```python
from build123d import *

# Parameters (mm, degrees)
SKETCH_1_R          = 5.25
EXTRUDE_1_DEPTH     = 5
CHAMFER_1_SIZE      = 0.4
SKETCH_2_R          = 1.2
CUT_EXTRUDE_1_DEPTH = 2.5
SKETCH_3_R          = 0.75
EXTRUDE_2_DEPTH     = 0.2
SKETCH_4_R          = 0.6
EXTRUDE_3_DEPTH     = 0.2
SKETCH_5_R          = 0.5
EXTRUDE_4_DEPTH     = 5.5
FILLET_1_R          = 0.1
SKETCH_6_R          = 2.5
EXTRUDE_5_DEPTH     = 1.7
EXTRUDE_6_DEPTH     = 1
SKETCH_8_R          = 0.7
CUT_EXTRUDE_2_DEPTH = 1
SKETCH_9_R          = 1.5
EXTRUDE_7_DEPTH     = 1.3
FILLET_2_R          = 0.2
CUT_EXTRUDE_3_DEPTH = 5.5


with BuildPart() as part:
    # 草图1 → 凸台-拉伸1 (new body)
    with BuildSketch(Plane.XY):
        Circle(SKETCH_1_R)
    extrude(amount=EXTRUDE_1_DEPTH)

    # 倒角1
    chamfer_1_edges = [part.edges().sort_by_distance(p)[0] for p in [
        (-5.25, 0, 5),
    ]]
    chamfer(chamfer_1_edges, length=CHAMFER_1_SIZE)

    # 草图2 → 切除-拉伸1 (cut)
    with BuildSketch(Plane.XY.offset(5)):
        with Locations((0, 3.25)):
            Circle(SKETCH_2_R)
        with Locations((3.090933678, 1.004305232)):
            Circle(SKETCH_2_R)
        with Locations((1.91030207, -2.629305232)):
            Circle(SKETCH_2_R)
        with Locations((-1.91030207, -2.629305232)):
            Circle(SKETCH_2_R)
        with Locations((-3.090933678, 1.004305232)):
            Circle(SKETCH_2_R)
    extrude(amount=-CUT_EXTRUDE_1_DEPTH, mode=Mode.SUBTRACT)

    # 草图3 → 凸台-拉伸2 (add)
    with BuildSketch(Plane.XY.offset(5)):
        Circle(SKETCH_3_R)
    extrude(amount=EXTRUDE_2_DEPTH)

    # 草图4 → 凸台-拉伸3 (add)
    with BuildSketch(Plane.XY.offset(5.2)):
        Circle(SKETCH_4_R)
    extrude(amount=EXTRUDE_3_DEPTH)

    # 草图5 → 凸台-拉伸4 (add)
    with BuildSketch(Plane.XY.offset(5.4)):
        Circle(SKETCH_5_R)
    extrude(amount=EXTRUDE_4_DEPTH)

    # 圆角1
    fillet_1_edges = [part.edges().sort_by_distance(p)[0] for p in [
        (-0.5, 0, 10.9),
    ]]
    fillet(fillet_1_edges, radius=FILLET_1_R)

    # 草图6 → 凸台-拉伸5 (add)
    with BuildSketch(Plane(origin=(0, 0, 0), x_dir=(-1, 0, 0), z_dir=(0, 0, -1))):
        Circle(SKETCH_6_R)
    extrude(amount=EXTRUDE_5_DEPTH)

    # 草图7 → 凸台-拉伸6 (add)
    with BuildSketch(Plane(origin=(0, 0, -1.7), x_dir=(-1, 0, 0), z_dir=(0, 0, -1))):
        with BuildLine():
            ThreePointArc((1.270195148, 3.576774791), (0, 4.6), (-1.270195148, 3.576774791))
            ThreePointArc((-1.270195148, 3.576774791), (-2.166553875, 1.259382495), (-3.725295111, -0.675583082))
            ThreePointArc((-3.725295111, -0.675583082), (-3.976336561, -2.287216952), (-2.455099963, -2.875625614))
            ThreePointArc((-2.455099963, -2.875625614), (0, -2.493198894), (2.455099963, -2.875625614))
            ThreePointArc((2.455099963, -2.875625614), (3.976336561, -2.287216952), (3.725295111, -0.675583082))
            ThreePointArc((3.725295111, -0.675583082), (2.166553875, 1.259382495), (1.270195148, 3.576774791))
        make_face()
    extrude(amount=EXTRUDE_6_DEPTH)

    # 草图8 → 切除-拉伸2 (cut)
    with BuildSketch(Plane(origin=(0, 0, -2.7), x_dir=(-1, 0, 0), z_dir=(0, 0, -1))):
        with Locations((0, 3.3)):
            Circle(SKETCH_8_R)
        with Locations((2.857883832, -1.65)):
            Circle(SKETCH_8_R)
        with Locations((-2.857883832, -1.65)):
            Circle(SKETCH_8_R)
    extrude(amount=-CUT_EXTRUDE_2_DEPTH, mode=Mode.SUBTRACT)

    # 草图9 → 凸台-拉伸7 (add)
    with BuildSketch(Plane(origin=(0, 0, -2.7), x_dir=(-1, 0, 0), z_dir=(0, 0, -1))):
        Circle(SKETCH_9_R)
    extrude(amount=EXTRUDE_7_DEPTH)

    # 圆角2
    fillet_2_edges = [part.edges().sort_by_distance(p)[0] for p in [
        (1.5, 0, -4),
    ]]
    fillet(fillet_2_edges, radius=FILLET_2_R)

    # 草图10 → 切除-拉伸3 (cut)
    with BuildSketch(Plane.XY.offset(10.9)):
        with BuildLine():
            Line((0.25, 0.441561144), (0.25, -0.441561144))
            ThreePointArc((0.25, -0.441561144), (0.50742117, 0), (0.25, 0.441561144))
        make_face()
    extrude(amount=-CUT_EXTRUDE_3_DEPTH, mode=Mode.SUBTRACT)


solid = part.part
```
Work out the finished part from the listing and answer in its coordinate system (mm). A direction names the side the tool comes from. Round coordinates to 2 decimals unless told otherwise and drop trailing zeros. Write each loop counter-clockwise with the first axis right and the second up, starting at its lowest first coordinate (ties: lowest second). Pieces come first, ordered by that corner, then holes. Notation, with made-up numbers: (57, 34.25) -> (102, 34.25) arc R20 cw to (102, 50.25) -> close; hole circle Ø9 at (67, -36). An arc over 180 degrees is marked (long way). Write each question's results on one line, items separated by ' | '.
Q1. Straight lines are drawn through the part: line 1 along Y through (x, z) = (2, 3); line 2 along Z through (x, y) = (0.5, 2.5); line 3 along Z through (x, y) = (0, -3). For each, find the intervals that lie inside material, in ascending order. Write a range as [from, to].
Data:
line 1: [-4.85, -3.83], [-1.43, 0.5], [1.5, 4.85] | line 2: [-2.7, -1.7], [0, 2.5] | line 3: [0, 5]
Q2. Determine the mould class of faces 4 (the flat face through (0, 0, -4)), 5 (the flat face through (-3, 1, 2.5)), 6 (the flat face through (0.25, 0, 8)) for opening direction X: released by +X, released by -X, zero draft, split by the parting line, or undercut.
Data:
face 4: zero draft | face 5: undercut | face 6: released by +X
Q3. Section A-A, the plane z = 6.5 is taken. Write down the section's boundary in (x, y).
Data:
outline: (0.25, -0.43) -> (0.25, 0.43) arc R0.5 ccw (long way) to start
Q4. Which of the six approach directions +Z, -Z, +X, -X, +Y, -Y give full straight-line access (tool end or side, diameter ignored) to faces 1 (the cylindrical face through (-1.357, -3.694, 3.768)), 2 (the cylindrical face through (-3.18, -2.27, -2.21)), 3 (the cylindrical face through (2.15, 1.29, -2.19))?
Data:
face 1: +Z | face 2: -Z | face 3: -Z, +X, +Y
Q5. Flat-ended cylindrical pins translate along their axes: P1, Ø2.5, axis at x = 0, y = 2.5, coming from the +Z side; P2, Ø1.4, axis at x = 3.09, y = 1, coming from the +Z side; P3, Ø1, axis at y = 4, z = 0, coming from the -X side; P4, Ø1.5, axis at y = 1.5, z = 9, coming from the +X side. Find the tip coordinate at first contact, or state that the pin passes through.
Data:
P1: z = 5 | P2: z = 2.5 | P3: x = -3.91 | P4: through
